Can you work these out from the model? Positions are in its coordinate system, mm. Face numbers are marked on the shaded views. A direction names the side the tool comes from. Coordinates: 2 decimals unless noted, no trailing zeros. Loops run counter-clockwise (first coordinate to the right, second up) from the corner with the lowest first, then second, coordinate; pieces in that order, holes last.
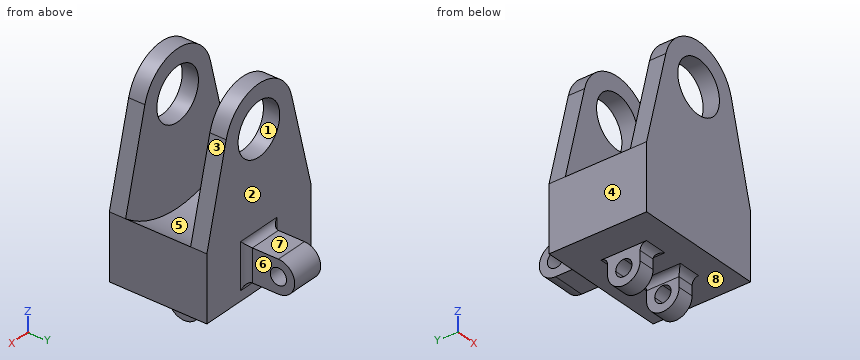
```python
from build123d import *

# Parameters (mm, degrees)
SKETCH1_R                = 16.51
SKETCH1_R_2              = 10.16
BOSS_EXTRUDE1_DEPTH      = 38.1
CUT_EXTRUDE1_START       = 6.35
SKETCH1_3_R              = 16.51
SKETCH1_3_R_2            = 10.16
CUT_EXTRUDE1_DEPTH       = 25.4
BOSS_EXTRUDE2_DEPTH      = 6.35
BOSS_EXTRUDE2_DEPTH_BACK = 6.35
BOSS_EXTRUDE3_START      = 6.35
BOSS_EXTRUDE3_DEPTH      = 6.35
BOSS_EXTRUDE4_START      = -12.7
BOSS_EXTRUDE4_DEPTH      = 6.35
FILLET1_R                = 2.54


with BuildPart() as part:
    # Sketch1 → Boss-Extrude1 (new body)
    # profile 1 of 4: a face of its own
    with BuildSketch(Plane(origin=(0, 0, 0), x_dir=(1, 0, 0), z_dir=(0, 1, 0))):
        with BuildLine():
            Line((-25.4, 57.934068682), (-25.4, 32.534068682))
            ThreePointArc((-25.4, 32.534068682), (0, 41.275), (25.4, 32.534068682))
            Line((25.4, 32.534068682), (25.4, 57.934068682))
            Line((25.4, 57.934068682), (-25.4, 57.934068682))
        make_face()
    # profile 2 of 4: a face of its own
    with BuildSketch(Plane(origin=(0, 0, 0), x_dir=(1, 0, 0), z_dir=(0, 1, 0))):
        with BuildLine():
            ThreePointArc((25.4, 32.534068682), (0, 41.275), (-25.4, 32.534068682))
            Line((-25.4, 32.534068682), (25.4, 32.534068682))
        make_face()
    # profile 3 of 4: a face of its own
    with BuildSketch(Plane(origin=(0, 0, 0), x_dir=(1, 0, 0), z_dir=(0, 1, 0))):
        with BuildLine():
            Line((25.4, 32.534068682), (-25.4, 32.534068682))
            Line((-25.4, 32.534068682), (-15.991186592, -4.106342823))
            ThreePointArc((-15.991186592, -4.106342823), (-2.069493823, 16.379783128), (16.51, 0))
            ThreePointArc((16.51, 0), (16.379783128, -2.069493823), (15.991186592, -4.106342823))
            Line((15.991186592, -4.106342823), (25.4, 32.534068682))
        make_face()
    # profile 4 of 4: a face of its own
    with BuildSketch(Plane(origin=(0, 0, 0), x_dir=(1, 0, 0), z_dir=(0, 1, 0))):
        Circle(SKETCH1_R)
        with Locations(Location((0, 0, 0), (0, 0, 90))):
            Circle(SKETCH1_R_2, mode=Mode.SUBTRACT)
    extrude(amount=BOSS_EXTRUDE1_DEPTH)

    # Sketch1_3 → Cut-Extrude1 (cut)
    # profile 1 of 3: a face of its own
    with BuildSketch(Plane(origin=(0, 0, 0), x_dir=(1, 0, 0), z_dir=(0, 1, 0)).offset(CUT_EXTRUDE1_START)):
        with BuildLine():
            Line((25.4, 32.534068682), (-25.4, 32.534068682))
            Line((-25.4, 32.534068682), (-15.991186592, -4.106342823))
            ThreePointArc((-15.991186592, -4.106342823), (-2.069493823, 16.379783128), (16.51, 0))
            ThreePointArc((16.51, 0), (16.379783128, -2.069493823), (15.991186592, -4.106342823))
            Line((15.991186592, -4.106342823), (25.4, 32.534068682))
        make_face()
    # profile 2 of 3: a face of its own
    with BuildSketch(Plane(origin=(0, 0, 0), x_dir=(1, 0, 0), z_dir=(0, 1, 0)).offset(CUT_EXTRUDE1_START)):
        with BuildLine():
            ThreePointArc((25.4, 32.534068682), (0, 41.275), (-25.4, 32.534068682))
            Line((-25.4, 32.534068682), (25.4, 32.534068682))
        make_face()
    # profile 3 of 3: a face of its own
    with BuildSketch(Plane(origin=(0, 0, 0), x_dir=(1, 0, 0), z_dir=(0, 1, 0)).offset(CUT_EXTRUDE1_START)):
        Circle(SKETCH1_3_R)
        with Locations(Location((0, 0, 0), (0, 0, 90))):
            Circle(SKETCH1_3_R_2, mode=Mode.SUBTRACT)
    extrude(amount=CUT_EXTRUDE1_DEPTH, mode=Mode.SUBTRACT)

    # Sketch3 → Boss-Extrude2 (add, two sides: drawn at the far end of the back side and taken through both)
    with BuildSketch(Plane.ZY.offset(-BOSS_EXTRUDE2_DEPTH_BACK)):
        with BuildLine():
            ThreePointArc((-51.584068682, 50.8), (-45.234068682, 44.45), (-38.884068682, 50.8))
            Line((-38.884068682, 50.8), (-42.059068682, 50.8))
            ThreePointArc((-42.059068682, 50.8), (-45.234068682, 47.625), (-48.409068682, 50.8))
            Line((-48.409068682, 50.8), (-51.584068682, 50.8))
        make_face()
        with BuildLine():
            Line((-42.059068682, 50.8), (-38.884068682, 50.8))
            ThreePointArc((-38.884068682, 50.8), (-45.234068682, 57.15), (-51.584068682, 50.8))
            Line((-51.584068682, 50.8), (-48.409068682, 50.8))
            ThreePointArc((-48.409068682, 50.8), (-45.234068682, 53.975), (-42.059068682, 50.8))
        make_face()
        with BuildLine():
            Line((-51.584068682, 38.1), (-45.234068682, 38.1))
            Line((-45.234068682, 38.1), (-38.884068682, 38.1))
            Line((-38.884068682, 38.1), (-38.884068682, 50.8))
            ThreePointArc((-38.884068682, 50.8), (-45.234068682, 44.45), (-51.584068682, 50.8))
            Line((-51.584068682, 50.8), (-51.584068682, 38.1))
        make_face()
    extrude(amount=BOSS_EXTRUDE2_DEPTH + BOSS_EXTRUDE2_DEPTH_BACK)

    # Sketch4 → Boss-Extrude3 (add)
    with BuildSketch(Plane.ZY.offset(BOSS_EXTRUDE3_START)):
        with BuildLine():
            Line((-64.284068682, 22.225), (-64.284068682, 25.4))
            ThreePointArc((-64.284068682, 25.4), (-70.634068682, 19.05), (-64.284068682, 12.7))
            Line((-64.284068682, 12.7), (-64.284068682, 15.875))
            ThreePointArc((-64.284068682, 15.875), (-67.459068682, 19.05), (-64.284068682, 22.225))
        make_face()
        with BuildLine():
            ThreePointArc((-64.284068682, 12.7), (-59.793940621, 14.559871939), (-57.934068682, 19.05))
            Line((-57.934068682, 19.05), (-61.109068682, 19.05))
            ThreePointArc((-61.109068682, 19.05), (-62.039004652, 16.80493597), (-64.284068682, 15.875))
            Line((-64.284068682, 15.875), (-64.284068682, 12.7))
        make_face()
        with BuildLine():
            Line((-61.109068682, 19.05), (-57.934068682, 19.05))
            ThreePointArc((-57.934068682, 19.05), (-59.793940621, 23.540128061), (-64.284068682, 25.4))
            Line((-64.284068682, 25.4), (-64.284068682, 22.225))
            ThreePointArc((-64.284068682, 22.225), (-62.039004652, 21.29506403), (-61.109068682, 19.05))
        make_face()
        with BuildLine():
            Line((-57.934068682, 12.7), (-57.934068682, 19.05))
            ThreePointArc((-57.934068682, 19.05), (-59.793940621, 14.559871939), (-64.284068682, 12.7))
            Line((-64.284068682, 12.7), (-57.934068682, 12.7))
        make_face()
        with BuildLine():
            ThreePointArc((-64.284068682, 25.4), (-59.793940621, 23.540128061), (-57.934068682, 19.05))
            Line((-57.934068682, 19.05), (-57.934068682, 25.4))
            Line((-57.934068682, 25.4), (-64.284068682, 25.4))
        make_face()
    extrude(amount=BOSS_EXTRUDE3_DEPTH)

    # Sketch4_3 → Boss-Extrude4 (add)
    with BuildSketch(Plane.ZY.offset(BOSS_EXTRUDE4_START)):
        with BuildLine():
            Line((-61.109068682, 19.05), (-57.934068682, 19.05))
            ThreePointArc((-57.934068682, 19.05), (-59.793940621, 23.540128061), (-64.284068682, 25.4))
            Line((-64.284068682, 25.4), (-64.284068682, 22.225))
            ThreePointArc((-64.284068682, 22.225), (-62.039004652, 21.29506403), (-61.109068682, 19.05))
        make_face()
        with BuildLine():
            Line((-64.284068682, 22.225), (-64.284068682, 25.4))
            ThreePointArc((-64.284068682, 25.4), (-70.634068682, 19.05), (-64.284068682, 12.7))
            Line((-64.284068682, 12.7), (-64.284068682, 15.875))
            ThreePointArc((-64.284068682, 15.875), (-67.459068682, 19.05), (-64.284068682, 22.225))
        make_face()
        with BuildLine():
            ThreePointArc((-64.284068682, 12.7), (-59.793940621, 14.559871939), (-57.934068682, 19.05))
            Line((-57.934068682, 19.05), (-61.109068682, 19.05))
            ThreePointArc((-61.109068682, 19.05), (-62.039004652, 16.80493597), (-64.284068682, 15.875))
            Line((-64.284068682, 15.875), (-64.284068682, 12.7))
        make_face()
        with BuildLine():
            ThreePointArc((-64.284068682, 25.4), (-59.793940621, 23.540128061), (-57.934068682, 19.05))
            Line((-57.934068682, 19.05), (-57.934068682, 25.4))
            Line((-57.934068682, 25.4), (-64.284068682, 25.4))
        make_face()
        with BuildLine():
            Line((-57.934068682, 12.7), (-57.934068682, 19.05))
            ThreePointArc((-57.934068682, 19.05), (-59.793940621, 14.559871939), (-64.284068682, 12.7))
            Line((-64.284068682, 12.7), (-57.934068682, 12.7))
        make_face()
    extrude(amount=BOSS_EXTRUDE4_DEPTH)

    # Fillet1
    fillet1_edges = [part.edges().sort_by_distance(p)[0] for p in [
        (0, 38.1, -38.884068682),
        (-6.35, 38.1, -45.234068682),
        (0, 38.1, -51.584068682),
        (6.35, 38.1, -45.234068682),
        (-9.525, 12.7, -57.934068682),
        (-9.525, 25.4, -57.934068682),
        (-6.35, 19.05, -57.934068682),
        (9.525, 25.4, -57.934068682),
        (9.525, 12.7, -57.934068682),
        (6.35, 19.05, -57.934068682),
    ]]
    fillet(fillet1_edges, radius=FILLET1_R)


solid = part.part
```
(1) I want a section at D-D on y = 20. Write out the boundary of the cut face in (x, z) (3 decimals), then the cut area to 3 significant figures.
Check values:
outline: (-25.4, -57.934) - (-12.7, -57.934) - (-12.7, -61.255) - (-6.35, -61.255) - (-6.35, -60.474) arc R2.54 cw to (-3.81, -57.934) - (3.81, -57.934) arc R2.54 cw to (6.35, -60.474) - (6.35, -61.255) - (12.7, -61.255) - (12.7, -57.934) - (25.4, -57.934) - (25.4, -32.534) arc R41.275 cw to (-25.4, -32.534) - close; (-12.7, -70.563) - (-6.35, -70.563) - (-6.35, -67.314) - (-12.7, -67.314) - close; (6.35, -70.563) - (12.7, -70.563) - (12.7, -67.314) - (6.35, -67.314) - close
area: 1,070 mm2
(2) I want a section at B-B on y = 5. Write out the boundary of the cut face in (x, z), then the cut area to 3 significant figures.
Check values:
outline: (-25.4, -57.93) - (25.4, -57.93) - (25.4, -32.53) - (15.99, 4.11) arc R16.51 ccw to (-15.99, 4.11) - (-25.4, -32.53) - close; hole circle Ø20.32 at (0, 0)
area: 2,780 mm2
(3) If we mould it in two halves opening along X, with no side actions, what happens to the marked faces 1, 2, 3 and 4? For each: released by +X, released by -X, zero draft, split by the parting line, or undercut.
Check values:
face 1: undercut
face 2: zero draft
face 3: released by +X
face 4: released by -X
(4) If I drill on probe 1 along Y at (x, z) = (13, 2.5); probe 2 along Y at (x, z) = (-20, -55.5), over which ranges is the centre line in solid material (lowest first)?
Check values:
probe 1: y = 0 to 6.35, 31.75 to 38.1
probe 2: y = 0 to 38.1
(5) I want a section at A-A on x = 0. Write out the boundary of the cut face in (y, z) (3 decimals).
Check values:
outline: (0, -57.934) - (38.1, -57.934) - (38.1, -54.124) arc R2.54 cw to (40.64, -51.584) - (50.8, -51.584) arc R6.35 ccw to (50.8, -38.884) - (40.64, -38.884) arc R2.54 cw to (38.1, -36.344) - (38.1, -10.16) - (31.75, -10.16) - (31.75, -41.275) - (6.35, -41.275) - (6.35, -10.16) - (0, -10.16) - close; (0, 10.16) - (6.35, 10.16) - (6.35, 16.51) - (0, 16.51) - close; (31.75, 10.16) - (38.1, 10.16) - (38.1, 16.51) - (31.75, 16.51) - close; hole circle Ø6.35 at (50.8, -45.234)
(6) Which directions (+Z, -Z, +X, -X, +Y, -Y) give clear straight access to the entire face, cutting with the end or side of a thin tool? Please do the marked faces 5, 6, 7 and 8.
Check values:
face 5: +Z
face 6: +Z, -Z, +X, +Y
face 7: +Z, +X, -X, +Y
face 8: -Z
(7) I'm going to push flat-ended pins straight in: pin 1 (2 mm diameter, centred on y = 33, z = 2.5, fed in from -X); pin 2 (4 mm diameter, centred on x = 9.5, z = -63, fed in from +Y); pin 3 (10 mm diameter, centred on y = 21, z = -61.5, fed in from +X); pin 4 (6 mm diameter, centred on y = 26.5, z = -25, fed in from -X). Where does each tip first touch, or does it pass through?
Check values:
pin 1: stops at x = -16.66
pin 2: stops at y = 25.4
pin 3: stops at x = 25.4
pin 4: passes through
(8) I want a section at C-C on z = 0. Write out the boundary of the cut face in (x, y), then the cut area to 3 significant figures.
Check values:
outline: (-17.05, 0) - (-10.16, 0) - (-10.16, 6.35) - (-17.05, 6.35) - close; (-17.05, 31.75) - (-10.16, 31.75) - (-10.16, 38.1) - (-17.05, 38.1) - close; (10.16, 0) - (17.05, 0) - (17.05, 6.35) - (10.16, 6.35) - close; (10.16, 31.75) - (17.05, 31.75) - (17.05, 38.1) - (10.16, 38.1) - close
area: 175 mm2
